from build123d import *

# Parameters (mm, degrees)
PAD003_DEPTH = 1.5
FILLET_R     = 12


with BuildPart() as sphere:
    # Sphere → Sphere (revolve)
    with BuildSketch(Plane(origin=(8, 26, 10.5), x_dir=(1, 0, 0), z_dir=(0, -1, 0))):
        with BuildLine():
            ThreePointArc((0, -10), (10, 0), (0, 10))
            Line((0, 10), (0, -10))
        make_face()
    revolve(axis=Axis((8, 26, 10.5), (0, 0, 1)))


with BuildPart() as clone_of_countersunk002:
    # Sketch007 → Revolution001 (revolve)
    with BuildSketch(Plane.YZ):
        Polygon((3.2, 0), (1.5, -1.7), (1.5, -10), (0, -10), (0, 0), align=None)
    revolve(axis=Axis((0, 0, 0), (0, 0, 1)))


with BuildPart() as clone_of_countersunk002_1:
    # Clone005 placement: moved
    add(clone_of_countersunk002.part.moved(Location((17.5, 21.5, 1.5))))


with BuildPart() as obj1:
    # Sketch → Pad003 (new body)
    with BuildSketch(Plane.XY):
        with BuildLine():
            ThreePointArc((19.061248, 16.249999), (19.574732, 16.450771), (20.06299, 16.706856))
            ThreePointArc((38.071883, 10.627711), (30.468372, 17.817422), (20.06299, 16.706856))
            ThreePointArc((38.071883, 10.627711), (39.189583, 10.018135), (40, 11))
            Line((40, 12), (40, 11))
            ThreePointArc((40, 12), (36.631728, 20.131728), (28.5, 23.5))
            Line((27.156854, 23.5), (28.5, 23.5))
            ThreePointArc((25.742641, 24.085786), (26.391487, 23.652241), (27.156854, 23.5))
            Line((25.742641, 24.085786), (17.414214, 32.414214))
            ThreePointArc((17.414214, 32.414214), (16.765367, 32.847759), (16, 33))
            Line((16, 33), (4.254623, 33))
            ThreePointArc((4.254623, 33), (3.341193, 32.779226), (2.629424, 32.165644))
            ThreePointArc((2.629424, 32.165644), (0.078439, 27.101717), (-0.8, 21.5))
            ThreePointArc((-0.8, 21.5), (-0.614027, 20.657798), (-0.090695, 19.972222))
            ThreePointArc((-0.090695, 19.972222), (9.000609, 15.617355), (19.061248, 16.249999))
        make_face()
    extrude(amount=PAD003_DEPTH)

    # Cut003: cut Clone of Countersunk002
    add(clone_of_countersunk002_1.part, mode=Mode.SUBTRACT)

    # Cut004: cut Sphere
    add(sphere.part, mode=Mode.SUBTRACT)

    # Fillet
    fillet_edges = [obj1.edges().sort_by_distance(p)[0] for p in [
        (3.641101, 26, 1.5),
    ]]
    fillet(fillet_edges, radius=FILLET_R)


solid = obj1.part
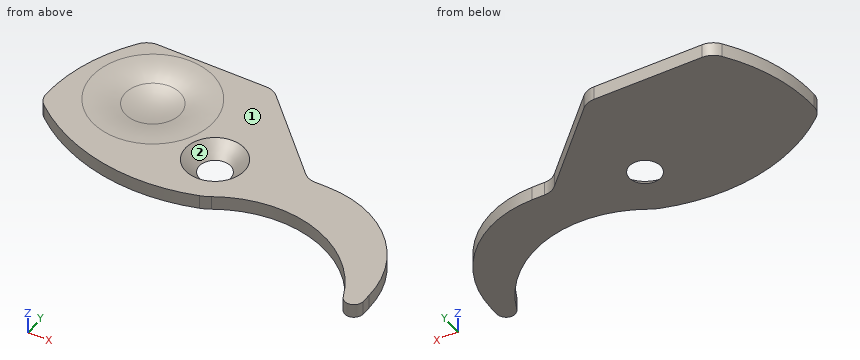
Work out the finished part from the listing and answer in its coordinate system (mm). Face numbers are marked on the shaded views. Give positions to 0.01 mm unless a question says otherwise; leave off trailing zeros. Order: outer loops, then holes, each group sorted by start corner. A loop starts at its lowest first (then second) coordinate and runs counter-clockwise, first axis right, second up. Notation, with made-up numbers: M -1,-34.5 L 27,-34.5 A30 ccw 27,0.5 Z; hole C 28.25,-14.5 d4. An arc over 180 degrees is marked long. Return JSON: item names as keys, results as strings.
Q1. Find section B-B, the plane x = 24.5. Write down the section's boundary in (y, z), and give its area (3 significant figures).
Answer below:
{"outline": "M 18.32,0 L 25.33,0 L 25.33,1.5 L 18.32,1.5 Z", "area": "10.5 mm^2"}
Q2. The mould has two halves that part along X. Classify the marked faces 1 and 2: pulls with the +X half, pulls with the -X half, needs draft (parallel to the pull), parting line crosses it, or undercut.
Answer below:
{"face 1": "needs draft", "face 2": "undercut"}
Q3. This flat-tipped pin is pushed along its axis until it touches: pin 1 (4 mm diameter, centred on x = 34.5, y = 21, fed in from -Z). Where does it stop, or does it pass through?
Answer below:
{"pin 1": "stops at z = 0"}
Q4. Find section C-C, the plane x = 34. Write down the section's boundary in (y, z), and give its area (3 significant figures).
Answer below:
{"outline": "M 15.95,0 L 22.1,0 L 22.1,1.5 L 15.95,1.5 Z", "area": "9.22 mm^2"}
Q5. Find section A-A, the plane z = 1.25. State how many separate pieces and enclosed holes the cut face has, and give its area (3 significant figures).
Answer below:
{"separate pieces": "1", "enclosed holes": "2", "area": "379 mm^2"}
Q6. Find the intervals of material crossed by line 1 along Y through (x, z) = (16, 0.2); line 2 along Y through (x, z) = (35.5, 0.25); line 3 along Y through (x, z) = (29, 0.45), in increasing order. Write a range as [from, to].
Answer below:
{"line 1": "y = [15.51, 20.33], [22.67, 33]", "line 2": "y = [14.62, 21.12]", "line 3": "y = [18.22, 23.49]"}
